Build history of the part. All positions in model axes, mm. A direction names the side the tool comes from. Give positions to 0.01 mm unless a question says otherwise; leave off trailing zeros. Write item = value, one per line. Start each with the question number.
Q1. Saw through at A-A, the plane x = 0. Give the number of separate pieces and of enclosed holes in the cut face, then the cut area to 3 significant figures.
Q2. Tool access for faces 1 (the face through (11.062, -2.078, 1.479)), 2 (the face through (9.54, 3, 3.02)): list every direction of +Z, -Z, +X, -X, +Y, -Y with a clear straight run to the whole face (end or side of a thin tool).
Q3. Wall check: line 1 (Y direction, x = 7, z = 5.5); line 2 (X direction, y = 26, z = 1); line 3 (Y direction, x = 10.5, z = 1). Give the ranges that are in metal, low to high.
Q4. Drop flat-ended pins along their axis: P1, Ø1.7, axis at x = -5.5, y = -3, coming from the +Z side; P2, Ø10, axis at x = 7, y = 15, coming from the +Z side; P3, Ø1.5, axis at y = 25, z = 6, coming from the -X side; P4, Ø3, axis at x = -5.2, y = -3, coming from the +Z side. Give the stop position or say it passes through.
from build123d import *

# Parameters (mm, degrees)
SKETCH1_R                = 50
SKETCH1_R_2              = 40
EXTRUDE_THIN1_DEPTH      = 10
SKETCH2_R                = 10
BOSS_EXTRUDE1_DEPTH      = 6
BOSS_EXTRUDE4_DEPTH      = 3
M2_CLEARANCE_HOLE1_D     = 2.4
M2_CLEARANCE_HOLE1_DEPTH = 10
M2_CLEARANCE_HOLE1_TIP   = 0.721032743
FILLET4_R                = 8
FILLET2_R                = 1
FILLET3_R                = 2
SKETCH7_R                = 4.6
CUT_EXTRUDE1_DEPTH       = 4
SKETCH8_R                = 1.75
CUT_EXTRUDE2_DEPTH       = 1.5
CIRPATTERN1_COUNT        = 3


with BuildPart() as part:
    # Sketch1 → Extrude-Thin1 (new body)
    with BuildSketch(Plane.XY):
        Circle(SKETCH1_R)
        Circle(SKETCH1_R_2, mode=Mode.SUBTRACT)
    extrude(amount=EXTRUDE_THIN1_DEPTH)



with BuildPart() as body_2:
    # Sketch2 → Boss-Extrude1 (new body)
    with BuildSketch(Plane.XY):
        Circle(SKETCH2_R)
    extrude(amount=BOSS_EXTRUDE1_DEPTH)


with BuildPart() as part_1:
    add(part.part)

    add(body_2.part)  # Boss-Extrude4 merges body 2
    # Sketch3 → Boss-Extrude4 (add)
    with BuildSketch(Plane.XY):
        with BuildLine():
            ThreePointArc((-3, 9.539392014), (-1.517576993, 9.884177258), (0, 10))
            Line((0, 10), (0, 40))
            ThreePointArc((0, 40), (-0.75, 39.992968132), (-1.499736305, 39.971875))
            Line((-1.499736305, 39.971875), (-3, 9.539392014))
        make_face()
        with BuildLine():
            Line((0, 40), (0, 10))
            ThreePointArc((0, 10), (1.517576993, 9.884177258), (3, 9.539392014))
            Line((3, 9.539392014), (1.499736305, 39.971875))
            ThreePointArc((1.499736305, 39.971875), (0.75, 39.992968132), (0, 40))
        make_face()
        with BuildLine():
            Line((6.761355821, -7.367772218), (33.866791034, -21.284747239))
            ThreePointArc((33.866791034, -21.284747239), (34.641016151, -20), (35.366527339, -18.687127761))
            Line((35.366527339, -18.687127761), (9.761355821, -2.171619796))
            ThreePointArc((9.761355821, -2.171619796), (8.660254038, -5), (6.761355821, -7.367772218))
        make_face()
        with BuildLine():
            ThreePointArc((-35.366527339, -18.687127761), (-34.641016151, -20), (-33.866791034, -21.284747239))
            Line((-33.866791034, -21.284747239), (-6.761355821, -7.367772218))
            ThreePointArc((-6.761355821, -7.367772218), (-8.660254038, -5), (-9.761355821, -2.171619796))
            Line((-9.761355821, -2.171619796), (-35.366527339, -18.687127761))
        make_face()
    extrude(amount=BOSS_EXTRUDE4_DEPTH)

    # M2 Clearance Hole1
    with Locations(Plane.XY.offset(6)):
        with Locations((0, 6), (-5.196152423, -3), (5.196152423, -3)):
            Hole(M2_CLEARANCE_HOLE1_D / 2, depth=M2_CLEARANCE_HOLE1_DEPTH)
            with Locations((0, 0, -(M2_CLEARANCE_HOLE1_DEPTH + M2_CLEARANCE_HOLE1_TIP / 2))):  # 118° drill point
                Cone(0, M2_CLEARANCE_HOLE1_D / 2, M2_CLEARANCE_HOLE1_TIP, mode=Mode.SUBTRACT)

    # Fillet4
    # the kernel refuses this fillet: 8 mm, written as the material it adds along each edge
    with BuildSketch(Plane(origin=(-3, 9.539392014, 0), x_dir=(-0.8901966603101863, -0.45557645458538654, 0), z_dir=(0, 0, 1)), Plane(origin=(9.761355821, -2.171619796, 0), x_dir=(0.05055754711810484, 0.9987211494853809, 0), z_dir=(0, 0, 1)), Plane(origin=(-6.761355821, -7.367772218, 0), x_dir=(0.8396391131920856, -0.5431446948999943, 0), z_dir=(0, 0, 1))) as fillet4_piece_1:
        with BuildLine():
            CenterArc((4.690930753, -7.886931421), FILLET4_R, 99.644427342, 50.431253784)
            Line((-2.242549971, -3.896086266), (0, 0))
            ThreePointArc((0, 0), (1.675332412, -0.141335724), (3.350664824, 0))
        make_face()
    extrude(amount=3)
    with BuildSketch(Plane(origin=(3, 9.539392014, 0), x_dir=(0.8901966603101863, -0.45557645458538637, 0), z_dir=(0, 0, 1)), Plane(origin=(6.761355821, -7.367772218, 0), x_dir=(-0.8396391131920875, -0.5431446948999916, 0), z_dir=(0, 0, 1)), Plane(origin=(-9.761355821, -2.171619796, 0), x_dir=(-0.05055754711810146, 0.9987211494853812, 0), z_dir=(0, 0, 1))) as fillet4_piece_2:
        with BuildLine():
            CenterArc((4.690930753, 7.886931421), FILLET4_R, 209.924318874, 50.431253784)
            Line((-2.242549971, 3.896086266), (0, 0))
            ThreePointArc((0, 0), (1.675332412, 0.141335724), (3.350664824, 0))
        make_face()
    extrude(amount=3)
    with BuildSketch(Plane(origin=(1.499736305, 39.971875, 0), x_dir=(0.04923830777365754, -0.9987870589107503, 0), z_dir=(0, 0, 1)), Plane(origin=(33.866791034, -21.284747239, 0), x_dir=(-0.8895941198746714, 0.4567519040840537, 0), z_dir=(0, 0, 1)), Plane(origin=(-35.366527339, -18.687127761, 0), x_dir=(0.8403558121010258, 0.542035154826719, 0), z_dir=(0, 0, 1))) as fillet4_piece_3:
        with BuildLine():
            CenterArc((9.974317113, 8), FILLET4_R, 159.003278938, 110.996721062)
            ThreePointArc((2.505509643, 10.866516174), (0.872211792, 5.521000489), (0, 0))
            Line((0, 0), (9.974317113, 0))
        make_face()
    extrude(amount=3)
    with BuildSketch(Plane(origin=(-1.499736305, 39.971875, 0), x_dir=(-0.04923830777365785, -0.9987870589107503, 0), z_dir=(0, 0, 1)), Plane(origin=(35.366527339, -18.687127761, 0), x_dir=(-0.8403558121010118, 0.5420351548267408, 0), z_dir=(0, 0, 1)), Plane(origin=(-33.866791034, -21.284747239, 0), x_dir=(0.8895941198746828, 0.4567519040840315, 0), z_dir=(0, 0, 1))) as fillet4_piece_4:
        with BuildLine():
            CenterArc((9.974317113, -8), FILLET4_R, 90, 110.996721062)
            ThreePointArc((2.505509643, -10.866516174), (0.872211792, -5.521000489), (0, 0))
            Line((0, 0), (9.974317113, 0))
        make_face()
    extrude(amount=3)

    # Fillet2
    fillet2_edges = [part_1.edges().sort_by_distance(p)[0] for p in [
        (-10, 0, 6),
    ]]
    fillet(fillet2_edges, radius=FILLET2_R)

    # Fillet3
    fillet3_edges = [part_1.edges().sort_by_distance(p)[0] for p in [
        (-50, 0, 0),
        (-50, 0, 10),
        (-40, 0, 10),
    ]]
    fillet(fillet3_edges, radius=FILLET3_R)

    # Sketch7 → Cut-Extrude1 (cut)
    with BuildSketch(Plane(origin=(0, 0, 0), x_dir=(-1, 0, 0), z_dir=(0, 0, -1))):
        Circle(SKETCH7_R)
    extrude(amount=-CUT_EXTRUDE1_DEPTH, mode=Mode.SUBTRACT)

    # Sketch8 → Cut-Extrude2 (cut)
    with BuildSketch(Plane.XY.offset(6)):
        with Locations((0, 6)):
            Circle(SKETCH8_R)
    cut_extrude2 = extrude(amount=-CUT_EXTRUDE2_DEPTH, mode=Mode.SUBTRACT)

    # CirPattern1: Cut-Extrude2 ×3 about axis
    cirpattern1_axis = Axis((0, 0, 0), (0, 0, 1))
    for i in range(1, CIRPATTERN1_COUNT):
        add(cut_extrude2.rotate(cirpattern1_axis, i * 360 / CIRPATTERN1_COUNT), mode=Mode.SUBTRACT)


solid = part_1.part
Report:
q1.separate_pieces = 3
q1.enclosed_holes = 0
q1.area = 352 mm2
q2.face_1 = +Z, -Z
q2.face_2 = +Z
q3.line_1 = -49.51 to -39.38, -6.95 to 6.95, 39.38 to 49.51
q3.line_2 = -42.39 to -30.4, -2.19 to 2.19, 30.4 to 42.39
q3.line_3 = -48.61 to -38.6, -9.29 to -0.98, 38.39 to 48.61
q4.P1 = through
q4.P2 = 3
q4.P3 = -43.73
q4.P4 = 4.5
